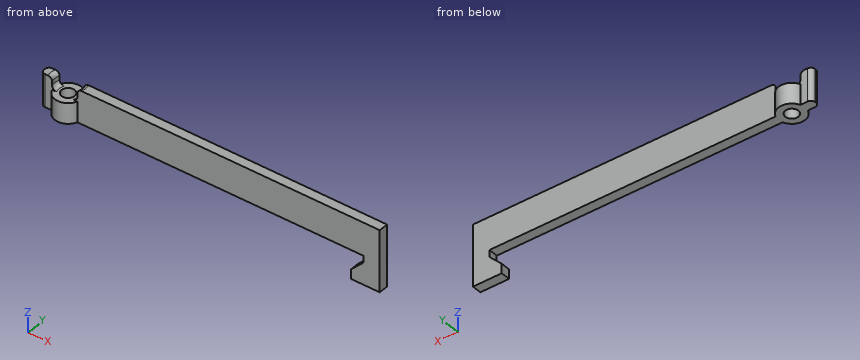
```python
from build123d import *

# Parameters (mm, degrees)
BOSS_EXTRUDE1_DEPTH = 2.3
SKETCH2_R           = 3.25
BOSS_EXTRUDE2_DEPTH = 8
SKETCH3_R           = 1.6
CUT_EXTRUDE1_DEPTH  = 8
CUT_EXTRUDE2_START  = -3
SKETCH4_R           = 3.25
CUT_EXTRUDE2_DEPTH  = 3
FILLET1_R           = 1
SKETCH5_W           = 5.3
SKETCH5_H           = 2.3
BOSS_EXTRUDE3_DEPTH = 3
CHAMFER1_SIZE       = 3


# Some blends are built 0.0001 mm under size
with BuildPart() as part:
    # Sketch1 → Boss-Extrude1 (new body)
    with BuildSketch(Plane(origin=(0, 0, 0), x_dir=(1, 0, 0), z_dir=(0, 1, 0))):
        Polygon((-78.5, 0), (0, 0), (0, 7), (4, 7), (4, -8), (-78.5, -8), align=None)
    extrude(amount=BOSS_EXTRUDE1_DEPTH)

    # Sketch2 → Boss-Extrude2 (add)
    with BuildSketch(Plane(origin=(0, 0, 0), x_dir=(-1, 0, 0), z_dir=(0, 0, -1))):
        with Locations((72.7, 1.076790216)):
            Circle(SKETCH2_R)
    extrude(amount=-BOSS_EXTRUDE2_DEPTH)

    # Sketch3 → Cut-Extrude1 (cut)
    with BuildSketch(Plane(origin=(0, 0, 0), x_dir=(-1, 0, 0), z_dir=(0, 0, -1))):
        with Locations((72.7, 1.076790216)):
            Circle(SKETCH3_R)
    extrude(amount=-CUT_EXTRUDE1_DEPTH, mode=Mode.SUBTRACT)

    # Sketch4 → Cut-Extrude2 (cut)
    with BuildSketch(Plane.XY.offset(8).offset(CUT_EXTRUDE2_START)):
        with Locations((-72.7, 1.076790216)):
            Circle(SKETCH4_R)
    extrude(amount=CUT_EXTRUDE2_DEPTH, mode=Mode.SUBTRACT)

    # Fillet1
    # the kernel refuses this fillet: 1 mm, written as the material it adds along each edge
    with BuildSketch(Plane(origin=(-72.7, 1.076790216, 5), x_dir=(-0.40375953104752016, 0.9148651491276113, 0), z_dir=(0.9148651491276113, 0.40375953104752016, 0))) as fillet1_piece_1_section:
        with BuildLine():
            CenterArc((3.25 - FILLET1_R, FILLET1_R), FILLET1_R, 270, 90)
            Line((3.25, FILLET1_R), (3.25, 0))
            Line((3.25, 0), (3.25 - FILLET1_R, 0))
        make_face()
    fillet1_piece_1 = revolve(axis=Axis((-72.7, 1.076790216, 5), (0, 0, 1)), revolution_arc=129.612934005, mode=Mode.PRIVATE)
    fillet1_piece_1 = split(fillet1_piece_1, bisect_by=Plane(origin=(-75.648358943, 2.3, 5.222958047), z_dir=(0, -1, 0)), keep=Keep.TOP, mode=Mode.PRIVATE)
    fillet1_piece_1 = split(fillet1_piece_1, bisect_by=Plane(origin=(-75.648358943, 0, 5.222958047), z_dir=(0, 1, 0)), keep=Keep.TOP, mode=Mode.PRIVATE)
    add(fillet1_piece_1)
    with BuildSketch(Plane(origin=(-72.7, 1.076790216, 5), x_dir=(0.44734781927350936, -0.8943600665231177, 0), z_dir=(-0.8943600665231177, -0.44734781927350936, 0))) as fillet1_piece_2_section:
        with BuildLine():
            CenterArc((3.25 - FILLET1_R, FILLET1_R), FILLET1_R, 270, 90)
            Line((3.25, FILLET1_R), (3.25, 0))
            Line((3.25, 0), (3.25 - FILLET1_R, 0))
        make_face()
    fillet1_piece_2 = revolve(axis=Axis((-72.7, 1.076790216, 5), (0, 0, 1)), revolution_arc=129.612934005, mode=Mode.PRIVATE)
    fillet1_piece_2 = split(fillet1_piece_2, bisect_by=Plane(origin=(-69.751641159, 2.3, 5.222958106), z_dir=(0, -1, 0)), keep=Keep.TOP, mode=Mode.PRIVATE)
    fillet1_piece_2 = split(fillet1_piece_2, bisect_by=Plane(origin=(-69.751641159, 0, 5.222958106), z_dir=(0, 1, 0)), keep=Keep.TOP, mode=Mode.PRIVATE)
    add(fillet1_piece_2)
    # the kernel refuses this fillet: 1 mm, written as the material it takes off along each edge
    with BuildSketch(Plane(origin=(-78.5, 2.3, 10.5), x_dir=(0, -1, 0), z_dir=(0, 0, -1)), Plane(origin=(-78.5, 0, 10.5), x_dir=(1, 0, 0), z_dir=(0, 0, -1))) as fillet1_2_piece_1:
        with BuildLine():
            CenterArc((FILLET1_R, -FILLET1_R), FILLET1_R, 90, 90)
            Line((0, -FILLET1_R), (0, 0))
            Line((0, 0), (FILLET1_R, 0))
        make_face()
    extrude(amount=13, mode=Mode.SUBTRACT)
    with BuildSketch(Plane(origin=(-72.7, 1.076790216, 8), x_dir=(-0.40375953104750745, 0.914865149127617, 0), z_dir=(0.914865149127617, 0.40375953104750745, 0))) as fillet1_2_piece_2:
        with BuildLine():
            CenterArc((3.25 + FILLET1_R, -FILLET1_R), FILLET1_R, 90, 90)
            Line((3.25, -FILLET1_R), (3.25, 0))
            Line((3.25, 0), (3.25 + FILLET1_R, 0))
        make_face()
    revolve(axis=Axis((-72.7, 1.076790216, 8), (0, 0, 1)), revolution_arc=129.612934005, mode=Mode.SUBTRACT)
    with BuildSketch(Plane(origin=(-72.7, 1.076790216, 8), x_dir=(0.44734781927345224, -0.8943600665231464, 7.1054273576009774e-15), z_dir=(-0.8943600665231464, -0.44734781927345224, 3.689898674328445e-15))) as fillet1_2_piece_3:
        with BuildLine():
            CenterArc((3.25 + FILLET1_R, -FILLET1_R), FILLET1_R, 90, 90)
            Line((3.25 + FILLET1_R, 0), (3.25, 0))
            Line((3.25, 0), (3.25, -FILLET1_R))
        make_face()
    revolve(axis=Axis((-72.7, 1.076790216, 8), (0, 0, 1)), revolution_arc=129.612934005, mode=Mode.SUBTRACT)

    # Sketch5 → Boss-Extrude3 (add)
    with BuildSketch(Plane.ZY):
        with Locations((-4.35, 1.15)):
            Rectangle(SKETCH5_W, SKETCH5_H)
    extrude(amount=BOSS_EXTRUDE3_DEPTH)

    # Chamfer1
    chamfer1_edges = [part.edges().sort_by_distance(p)[0] for p in [
        (-3, 1.15, -1.7),
    ]]
    chamfer(chamfer1_edges, length=CHAMFER1_SIZE - 0.0001)  # a hair under: the kernel refuses the full size


solid = part.part
```
CAD build for the part. Positions are in the model's coordinates, mm. Round coordinates to 2 decimals unless told otherwise and drop trailing zeros. Write each loop counter-clockwise with the first axis right and the second up, starting at its lowest first coordinate (ties: lowest second). Pieces come first, ordered by that corner, then holes. Notation, with made-up numbers: (78.5, -27) - (89.5, -27) arc R15 cw to (89.5, -19) - close; hole circle Ø10 at (89, 87). An arc over 180 degrees is marked (long way). Return JSON: item names as keys, results as strings. Group by question number.
Item 1: Band-saw the part on A-A on x = -72.7. List the corners of the cut face in (y, z), plus the area to 3 significant figures.
Item 2: Band-saw the part on B-B on z = 3.75. List the corners of the cut face in (x, y), plus the area to 3 significant figures.
Item 3: Flat gauge pins, fed straight in: pin 1 Ø0.9 at (x, z) = (-76.5, 5.5) entering from +Y; pin 2 Ø1.5 at (x, z) = (-53, 1) entering from -Y; pin 3 Ø3 at (x, y) = (-49, 1) entering from -Z; pin 4 Ø1 at (x, y) = (-17.5, -1) entering from -Z. Where does each tip first touch, or does it go through?
Item 4: Band-saw the part on C-C on z = -5.5. List the corners of the cut face in (x, y).
Item 5: Probe probe 1 along Y at (x, z) = (-72.7, 1.8); probe 2 along Z at (x, y) = (-31, 1); probe 3 along X at (y, z) = (1.5, -1.5). List the from-to ranges inside material, lowest first.
Resolved:
{
 "1": {"outline": "(-2.17, 0) - (-0.52, 0) - (-0.52, 5) - (-2.17, 5) - close; (2.68, 0) - (4.33, 0) - (4.33, 5) - (2.68, 5) - close", "area": "16.5 mm²"},
 "2": {"outline": "(-78.5, 1) arc R1 ccw to (-77.5, 0) - (-75.77, 0) arc R3.25 ccw to (-69.63, 0) - (4, 0) - (4, 2.3) - (-69.69, 2.3) arc R3.25 ccw to (-75.71, 2.3) - (-77.5, 2.3) arc R1 ccw to (-78.5, 1.3) - close; hole circle Ø3.2 at (-72.7, 1.08)", "area": "200 mm²"},
 "3": {"pin 1": "stops at y = 2.3", "pin 2": "stops at y = 0", "pin 3": "stops at z = 0", "pin 4": "passes through"},
 "4": {"outline": "(-3, 0) - (4, 0) - (4, 2.3) - (-3, 2.3) - close"},
 "5": {"probe 1": "y = -2.17 to -0.52, 2.68 to 4.33", "probe 2": "z = 0 to 8", "probe 3": "x = 0 to 4"}
}
